Source: CAD feature listing. Evaluate the final solid. Frame: model axes, mm. Round coordinates to 2 decimals unless told otherwise and drop trailing zeros. Order: outer loops, then holes, each group sorted by start corner. A loop starts at its lowest first (then second) coordinate and runs counter-clockwise, first axis right, second up.
Autodesk Inventor part; units mm, degrees
ref_plane "Work Plane3" through (6, 0, 0) normal (1, 0, 0) x (0, 1, 0)
ref_plane "XZ Plane" through (0, 0, 0) normal (0, 1, 0) x (-1, 0, 0)
ref_plane "XY Plane" through (0, 0, 0) normal (0, 0, 1) x (1, 0, 0)
sketch "Sketch1" plane through (0, 0, 0) normal (0, 1, 0) x (-1, 0, 0)
  circle A0 centre (0, 0) radius 5
  circle A1 centre (0, 0) radius 6
  dimension "d1" = 1
  dimension "d34" = 10
extrude "Extrusion1" add sketch "Sketch1" along normal blind 271.1467
ref_plane "Work Plane3" through (6, 0, 0) normal (1, 0, 0) x (0, 1, 0)
sketch "Sketch2" plane through (6, 0, 0) normal (1, 0, 0) x (0, 1, 0)
  line L0 (0, -6) -> (271.1467, -6)
  line L1 (0, 6) -> (271.1467, 6)
  line L2 (271.1467, -6) -> (271.1467, 6)
  line L3 (-54.2293, 0) -> (325.3761, 0)
  point P0 (0, 0)
  point P1 (10, 0)
  point P2 (271.1467, 0)
  dimension "d20" = 10
hole "Hole1" at (6, 10, 0) direction (-1, 0, 0) diameter 6 end up to surface
sketch "Sketch3" plane through (6, 0, 0) normal (1, 0, 0) x (0, 1, 0)
  line L0 (-54.2293, 0) -> (325.3761, 0)
  line L1 (271.1467, -6) -> (271.1467, 6)
  line L2 (236.1467, 6) -> (271.1467, 6)
  line L3 (271.1467, 6) -> (271.1467, -6)
  line L4 (271.1467, -6) -> (236.1467, -6)
  line L5 (236.1467, -6) -> (236.1467, 6)
  point P0 (0, 0)
  point P1 (245.6467, 0)
  point P2 (263.6467, 0)
  dimension "d22" = 7.5
  dimension "d23" = 18
  dimension "d24" = 35
extrude "Extrusion2" cut sketch "Sketch3" against normal blind 7
hole "Hole3" at (6, 263.6467, 0) at (6, 245.6467, 0) direction (-1, 0, 0) diameter 5 end through all
equation "\"d1\" = pipe_thickness"
equation "\"d34\" = pipe_inner_diameter"
equation "\"d2\" = pipe_length"
equation "\"d24\" = bar_connection"
equation "\"d25\" = pipe_cutout"
equation "\"pipe_length\" = connector_min_length - bar_connection"
equation "\"alfa\" = 45deg"
equation "\"bar_connection\" = 35"
equation "\"pipe_cutout\" = 7"
equation "\"pipe_inner_diameter\" = 10"
equation "\"pipe_thickness\" = 1"
equation "\"pipe_outer_diameter\" = pipe_inner_diameter + 2 * pipe_thickness"
properties part number "pipe" material "Aluminum 6061"
1. Section B-B on y = 223.5. Return loops of the section in (x, z), plus the area to 3 significant figures.
2. Line query: line 1 along Y through (x, z) = (-5.2, 0); line 2 along X through (y, z) = (200.5, 0); line 3 along Z through (x, y) = (0.5, 139). Output: solid intervals per line, ascending.
3. First-contact query: pin 1 (5 mm diameter, centred on x = 3.5, z = 4, fed in from +Y); pin 2 (3 mm diameter, centred on y = 208.5, z = 3.5, fed in from -X); pin 3 (5 mm diameter, centred on y = 10, z = 0, fed in from +X). Flat tips, straight axial feed; report the tip coordinate or a pass-through.
4. Section A-A on z = 0. Return loops of the section in (x, y).
5. Section C-C on y = 253.5. Return loops of the section in (x, z), plus the area to 3 significant figures.
6. Section D-D on y = 10. Return loops of the section in (x, z), plus the area to 3 significant figures.
7. Pull-direction query (Y, two-part tool) for faces 1 (the face through (4.99, 7.97, 2.21)), 2 (the face through (-5.177, 245.537, 2.498)), 3 (the face through (4, 0, 4)), 4 (the face through (5.1, 236.147, -1.4)); classes: released by +Y, released by -Y, zero draft, split by the parting line, or undercut.
Result:
1. outline: circle Ø12 at (0, 0); hole circle Ø10 at (0, 0)
1. area: 34.6 mm2
2. line 1: y = 0 to 243.15, 248.15 to 261.15, 266.15 to 271.15
2. line 2: x = -6 to -5, 5 to 6
2. line 3: z = -5.98 to -4.97, 4.97 to 5.98
3. pin 1: stops at y = 236.15
3. pin 2: stops at x = -5.66
3. pin 3: stops at x = -4.33
4. outline: (-6, 0) - (-5, 0) - (-5, 243.15) - (-6, 243.15) - close; (-6, 248.15) - (-5, 248.15) - (-5, 261.15) - (-6, 261.15) - close; (-6, 266.15) - (-5, 266.15) - (-5, 271.15) - (-6, 271.15) - close; (5, 0) - (6, 0) - (6, 7) - (5, 7) - close; (5, 13) - (6, 13) - (6, 236.15) - (5, 236.15) - close
5. outline: (-1, -5.92) - (-1, -4.9) arc R5 cw to (-1, 4.9) - (-1, 5.92) arc R6 ccw to start
5. area: 15.3 mm2
6. outline: (4, -3) arc R5 cw (long way) to (4, 3) - (5.2, 3) arc R6 ccw (long way) to (5.2, -3) - close
6. area: 28.2 mm2
7. face 1: undercut
7. face 2: undercut
7. face 3: released by -Y
7. face 4: released by +Y
